from build123d import *

# Parameters (mm, degrees)
BOSS_EXTRUDE1_DEPTH   = 4.7625
F_6_CLEARANCE_HOLE1_D = 4.3053
SKETCH4_R             = 4.7625
SKETCH4_R_2           = 9.525
CUT_EXTRUDE1_DEPTH    = 5.7625


with BuildPart() as part:
    # Sketch1 → Boss-Extrude1 (new body)
    with BuildSketch(Plane.XY):
        with BuildLine():
            Line((133.2865, 94.45625), (12.7635, 94.45625))
            ThreePointArc((12.7635, 94.45625), (11.685869265, 94.009880735), (11.2395, 92.93225))
            Line((11.2395, 92.93225), (11.2395, 80.9625))
            ThreePointArc((11.2395, 80.9625), (9.379628061, 76.472371939), (4.8895, 74.6125))
            Line((4.8895, 74.6125), (2.31775, 74.6125))
            ThreePointArc((2.31775, 74.6125), (1.240119265, 74.166130735), (0.79375, 73.0885))
            Line((0.79375, 73.0885), (0.79375, 22.1615))
            ThreePointArc((0.79375, 22.1615), (1.240119265, 21.083869265), (2.31775, 20.6375))
            Line((2.31775, 20.6375), (4.8895, 20.6375))
            ThreePointArc((4.8895, 20.6375), (9.379628061, 18.777628061), (11.2395, 14.2875))
            Line((11.2395, 14.2875), (11.2395, 2.31775))
            ThreePointArc((11.2395, 2.31775), (11.685869265, 1.240119265), (12.7635, 0.79375))
            Line((12.7635, 0.79375), (133.2865, 0.79375))
            ThreePointArc((133.2865, 0.79375), (134.364130735, 1.240119265), (134.8105, 2.31775))
            Line((134.8105, 2.31775), (134.8105, 14.2875))
            ThreePointArc((134.8105, 14.2875), (136.670371939, 18.777628061), (141.1605, 20.6375))
            Line((141.1605, 20.6375), (143.73225, 20.6375))
            ThreePointArc((143.73225, 20.6375), (144.809880735, 21.083869265), (145.25625, 22.1615))
            Line((145.25625, 22.1615), (145.25625, 73.0885))
            ThreePointArc((145.25625, 73.0885), (144.809880735, 74.166130735), (143.73225, 74.6125))
            Line((143.73225, 74.6125), (141.1605, 74.6125))
            ThreePointArc((141.1605, 74.6125), (136.670371939, 76.472371939), (134.8105, 80.9625))
            Line((134.8105, 80.9625), (134.8105, 92.93225))
            ThreePointArc((134.8105, 92.93225), (134.364130735, 94.009880735), (133.2865, 94.45625))
        make_face()
    extrude(amount=BOSS_EXTRUDE1_DEPTH)

    # #6 Clearance Hole1 (through all)
    with Locations(Plane.XY.offset(4.7625)):
        with Locations((46.99, 82.55), (97.79, 82.55), (85.725, 9.525), (46.99, 9.525)):
            Hole(F_6_CLEARANCE_HOLE1_D / 2)

    # Sketch4 → Cut-Extrude1 (cut, through all)
    with BuildSketch(Plane.XY.offset(4.7625)):
        with Locations((73.025, 68.326)):
            Circle(SKETCH4_R)
        with Locations((104.775, 21.59)):
            Circle(SKETCH4_R)
        with Locations((30.988, 66.675)):
            Circle(SKETCH4_R_2)
        with Locations((113.03, 66.675)):
            Circle(SKETCH4_R_2)
        with Locations((31.242, 20.955)):
            Circle(SKETCH4_R_2)
        with Locations((64.5795, 20.955)):
            Circle(SKETCH4_R_2)
    extrude(amount=-CUT_EXTRUDE1_DEPTH, mode=Mode.SUBTRACT)


solid = part.part
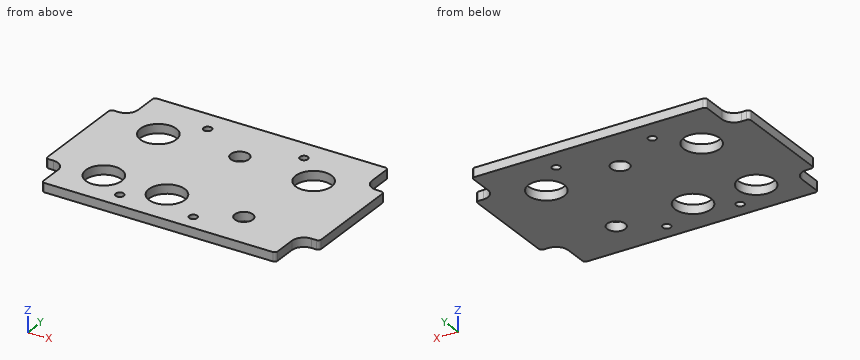
Verification items for the finished model (mm, model axes). Coordinates: 2 decimals unless noted, no trailing zeros. Order: outer loops, then holes, each group sorted by start corner. A loop starts at its lowest first (then second) coordinate and runs counter-clockwise, first axis right, second up. Notation, with made-up numbers: M -12.75,38 L 27.25,38 A25 cw 27.25,53 Z; hole C 61.25,23.5 d9. An arc over 180 degrees is marked long. One line per item, written item: value. Start each with the question number.
Item 1: Sectioned sample at C-C on x = 25.5. Record the cut outline in (y, z).
Item 2: Depth check by flat-ended pin: P1, Ø3.5, axis at x = 97.79, y = 82.55, coming from the +Z side; P2, Ø2.5, axis at y = 10.5, z = 2.5, coming from the -X side; P3, Ø2, axis at x = 142, z = 1.5, coming from the -Y side; P4, Ø1.3, axis at x = 4, z = 2, coming from the +Y side. Enter the tip coordinate at first touch or a pass-through.
Item 3: Sectioned sample at A-A on x = 97.79. Record the cut outline in (y, z).
Item 4: Thickness scan on probe 1 along X at (y, z) = (66.5, 2); probe 2 along X at (y, z) = (9, 0.55); probe 3 along X at (y, z) = (70.5, 2.7). Record the ranges inside material, lowest first.
Item 5: Sectioned sample at D-D on z = 2.7. Give the number of separate pieces and of enclosed holes in the cut face, then the cut area to 3 significant figures.
Item 6: Sectioned sample at B-B on y = 82.55. Record the cut outline in (x, z), then the cut area to 4 significant figures.
Calculated:
1. outline: M 0.79,0 L 13.36,0 L 13.36,4.76 L 0.79,4.76 Z; M 28.55,0 L 58.89,0 L 58.89,4.76 L 28.55,4.76 Z; M 74.46,0 L 94.46,0 L 94.46,4.76 L 74.46,4.76 Z
2. P1: through
2. P2: x = 11.24
2. P3: y = 20.64
2. P4: y = 74.61
3. outline: M 0.79,0 L 80.4,0 L 80.4,4.76 L 0.79,4.76 Z; M 84.7,0 L 94.46,0 L 94.46,4.76 L 84.7,4.76 Z
4. probe 1: 0.79 to 21.46, 40.51 to 68.63, 77.42 to 103.51, 122.55 to 145.26
4. probe 2: 11.24 to 44.9, 49.08 to 83.64, 87.81 to 134.81
4. probe 3: 0.79 to 22.26, 39.71 to 68.79, 77.26 to 104.31, 121.75 to 145.26
5. separate pieces: 1
5. enclosed holes: 10
5. area: 11,400 mm^2
6. outline: M 11.24,0 L 44.84,0 L 44.84,4.76 L 11.24,4.76 Z; M 49.14,0 L 95.64,0 L 95.64,4.76 L 49.14,4.76 Z; M 99.94,0 L 134.81,0 L 134.81,4.76 L 99.94,4.76 Z
6. area: 547.5 mm^2
